Can you work these out from the model? Positions are in its coordinate system, mm. Face numbers are marked on the shaded views. A direction names the side the tool comes from. Round coordinates to 2 decimals unless told otherwise and drop trailing zeros. Loops run counter-clockwise (first coordinate to the right, second up) from the corner with the lowest first, then second, coordinate; pieces in that order, holes last. Notation, with made-up numbers: M 83,67.5 L 120,67.5 A8 cw 120,76.5 Z; hole C 38,-3.75 d1. An arc over 180 degrees is marked long. Use a Markdown table: item, result. Add a question column.
```python
from build123d import *

# Parameters (mm, degrees)
BASENUTSKE_R  = 8.75
BASENUT_DEPTH = 30
COLLARSKE_W   = 6
COLLARSKE_H   = 9.75
FILLET_2_R    = 0.5


with BuildPart() as part:
    # BaseNutSke → BaseNut (new body)
    with BuildSketch(Plane.XY):
        Polygon((15, 8.660254038), (15, -8.660254038), (0, -17.320508076), (-15, -8.660254038), (-15, 8.660254038), (0, 17.320508076), align=None)
        Circle(BASENUTSKE_R, mode=Mode.SUBTRACT)
    extrude(amount=-BASENUT_DEPTH)

    # CollarSke → Collar (revolve)
    with BuildSketch(Plane(origin=(0, 0, 0), x_dir=(0, 0, -1), z_dir=(1, 0, 0)), mode=Mode.PRIVATE) as collar_sk:
        with Locations((27, 13.625)):
            Rectangle(COLLARSKE_W, COLLARSKE_H)
    revolve(collar_sk.sketch.rotate(Axis((0, 0, 0), (0, 0, -1)), 90), axis=Axis((0, 0, 0), (0, 0, -1)))

    # Sketch3 → Chamfer 2 (revolve, cut)
    with BuildSketch(Plane(origin=(0, 0, 0), x_dir=(0, 0, -1), z_dir=(1, 0, 0))):
        Polygon((2, 30.020508076), (-12.7, 30.020508076), (-12.7, 15), (0, 15), (2, 17.320508076), align=None)
    revolve(axis=Axis((0, 0, 0), (0, 0, -1)), mode=Mode.SUBTRACT)

    # Sketch5 → EndChamfer (revolve, cut)
    with BuildSketch(Plane(origin=(0, 0, 0), x_dir=(0, 0, -1), z_dir=(1, 0, 0)), mode=Mode.PRIVATE) as endchamfer_sk:
        Polygon((29.9746, 10), (29.011814635, 8.625), (30.0254, 8.625), (30.0254, 10), align=None)
        Polygon((-0.0508, 10), (0, 10), (0.962785365, 8.625), (-0.0508, 8.625), align=None)
    revolve(endchamfer_sk.sketch.rotate(Axis((0, 0, -25.037505729), (0, 0, -1)), 90), axis=Axis((0, 0, -25.037505729), (0, 0, -1)), mode=Mode.SUBTRACT)

    # Fillet 2
    fillet_2_edges = [part.edges().sort_by_distance(p)[0] for p in [
        (7.5, 12.990381057, -24),
        (-7.5, 12.990381057, -24),
        (-15, 0, -24),
        (-7.5, -12.990381057, -24),
        (7.5, -12.990381057, -24),
        (15, 0, -24),
    ]]
    fillet(fillet_2_edges, radius=FILLET_2_R)


solid = part.part
```
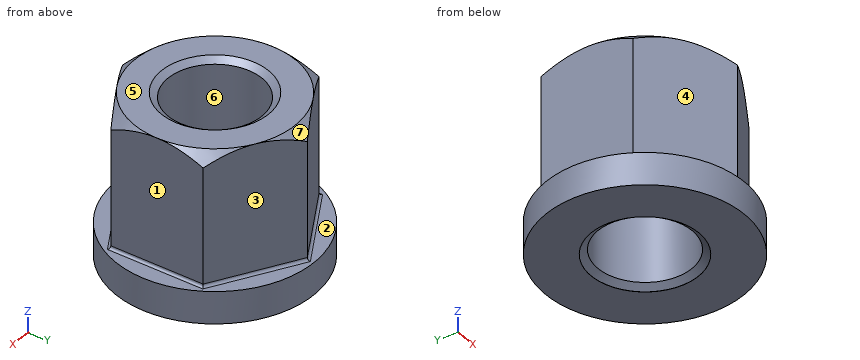
(1) Suppose I cut it at B-B on z = -28. List the corners of the cut face in (x, y) for me.
(2) On a 3-axis mill with a long thin cutter (end or side, diameter ignored), from which of +Z, -Z, +X, -X, +Y, -Y can I reach the whole of each face in a straight line? I mean the marked faces 1, 2, 3 and 4. Say none if no direction works.
(3) Suppose I cut it at A-A on z = -3. List the corners of the cut face in (x, y) for me.
(4) I'm going to push flat-ended pins straight in: pin 1 (1 mm diameter, centred on y = 2.5, z = -25.5, fed in from +X); pin 2 (8.5 mm diameter, centred on y = 0, z = -9, fed in from -X); pin 3 (3 mm diameter, centred on x = 7, z = -4, fed in from -Y). Where does each tip first touch, or does it pass through?
(5) If I drill on probe 1 along Y at (x, z) = (0, -16.25); probe 2 along Z at (x, y) = (-2, -17); probe 3 along Y at (x, z) = (-14.5, -22), over which ranges is the centre line in solid material (lowest first)? Write a range as [from, to].
(6) Thinking about a two-plate mould opening in Y: for the marked faces 5, 6 and 7, which applies, released by +Y, released by -Y, zero draft, split by the parting line, or undercut?
Results below:
| question | item | result |
|---|---|---|
| 1 | outline | C 0,0 d37; hole C 0,0 d17.5 |
| 2 | face 1 | +Z, +X, +Y, -Y |
| 2 | face 2 | +Z |
| 2 | face 3 | +Z, +X, +Y |
| 2 | face 4 | +Z, -X, -Y |
| 3 | outline | M -15,-8.66 L 0,-17.32 L 15,-8.66 L 15,8.66 L 0,17.32 L -15,8.66 Z; hole C 0,0 d17.5 |
| 4 | pin 1 | stops at x = 18.39 |
| 4 | pin 2 | stops at x = -15 |
| 4 | pin 3 | stops at y = -14.15 |
| 5 | probe 1 | y = [-17.32, -8.75], [8.75, 17.32] |
| 5 | probe 2 | z = [-30, -24] |
| 5 | probe 3 | y = [-8.95, 8.95] |
| 6 | face 5 | zero draft |
| 6 | face 6 | undercut |
| 6 | face 7 | released by +Y |
